CAD build for the part. Positions are in the model's coordinates, mm. A direction names the side the tool comes from. Round coordinates to 2 decimals unless told otherwise and drop trailing zeros. Answer as a JSON object with one key per item and string values.
```python
from build123d import *

# Parameters (mm, degrees)
SKETCH2_R          = 9.525
CUT_EXTRUDE1_DEPTH = 148.442344892
SKETCH3_R          = 6.35
CUT_EXTRUDE2_DEPTH = 3.81
CIRPATTERN1_COUNT  = 15
FILLET1_R          = 1.27


with BuildPart() as part:
    # Sketch1 → Revolve1 (revolve)
    with BuildSketch(Plane.XY, mode=Mode.PRIVATE) as revolve1_sk:
        with BuildLine():
            Line((0, 0), (50.8, 0))
            ThreePointArc((50.8, 0), (77.507770873, 6.756373885), (97.79, 25.4))
            Line((97.79, 25.4), (97.79, 3.81))
            Line((97.79, 3.81), (78.74, 3.81))
            Line((78.74, 3.81), (78.74, 0))
            Line((78.74, 0), (101.6, 0))
            Line((101.6, 0), (101.6, 33.077561287))
            Line((101.6, 33.077561287), (97.79, 33.077561287))
            ThreePointArc((97.79, 33.077561287), (78.479641633, 11.725205481), (50.8, 3.81))
            Line((50.8, 3.81), (0, 3.81))
            Line((0, 3.81), (0, 0))
        make_face()
    revolve(revolve1_sk.sketch.rotate(Axis((0, 0, 0), (0, 1, 0)), 90), axis=Axis((0, 0, 0), (0, 1, 0)))

    # Sketch2 → Cut-Extrude1 (cut, through all)
    with BuildSketch(Plane.XZ):
        with Locations(Location((-22.225, 0, 0), (0, 0, 270))):
            Circle(SKETCH2_R)
        with Locations(Location((22.225, 0, 0), (0, 0, 270))):
            Circle(SKETCH2_R)
    extrude(amount=-CUT_EXTRUDE1_DEPTH, mode=Mode.SUBTRACT)

    # Sketch3 → Cut-Extrude2 (cut)
    with BuildSketch(Plane.XZ):
        with Locations(Location((-88.9, 0, 0), (0, 0, 270))):
            Circle(SKETCH3_R)
    cut_extrude2 = extrude(amount=-CUT_EXTRUDE2_DEPTH, mode=Mode.SUBTRACT)

    # CirPattern1: Cut-Extrude2 ×15 about axis
    cirpattern1_axis = Axis((0, 0, 0), (0, 1, 0))
    for i in range(1, CIRPATTERN1_COUNT):
        add(cut_extrude2.rotate(cirpattern1_axis, i * 360 / CIRPATTERN1_COUNT), mode=Mode.SUBTRACT)

    # Fillet1
    fillet1_edges = [part.edges().sort_by_distance(p)[0] for p in [
        (0, 3.81, 78.74),
        (0, 3.81, 97.79),
    ]]
    fillet(fillet1_edges, radius=FILLET1_R)


solid = part.part
```
Item 1: 3-axis set-ups, long thin cutter, end or side, ignore diameter. For faces 1 (the flat face through (57, 3.81, 58)), 2 (the cylindrical face through (8.57, 1.88, -94.72)), 3 (the flat face through (-83, 33.078, 53)): which of +Z, -Z, +X, -X, +Y, -Y reach the whole face in a straight line?
Worked answers:
{"face 1": "none", "face 2": "-Y", "face 3": "+Z, -Z, +X, -X, +Y"}
Item 2: Wall check: line 1 along X through (y, z) = (19.5, -63.5); line 2 along X through (y, z) = (23, -46); line 3 along Y through (x, z) = (10, -44.5). Give the ranges that are in metal, low to high. Write a range as [from, to].
Worked answers:
{"line 1": "x = [-79.31, -74.37], [-68.42, -61.17], [61.17, 68.42], [74.37, 79.31]", "line 2": "x = [-90.59, -86.3], [-84.41, -78.88], [78.88, 84.41], [86.3, 90.59]", "line 3": "y = [0, 3.81]"}
Item 3: Drop flat-ended pins along their axis: pin 1 Ø16.5 at (x, z) = (44.45, -76.99) entering from -Y; pin 2 Ø11.5 at (x, z) = (86.96, 18.48) entering from +Y; pin 3 Ø1.5 at (x, y) = (36, 9.5) entering from +Z; pin 4 Ø10 at (y, z) = (29, 34.5) entering from -X. Give the stop position or say it passes through.
Worked answers:
{"pin 1": "stops at y = 0", "pin 2": "stops at y = 27.56", "pin 3": "stops at z = 95.29", "pin 4": "stops at x = -97.22"}
Item 4: Saw through at A-A on z = 0. State how many separate pieces and enclosed holes the cut face has, and give its area (3 significant figures).
Worked answers:
{"separate pieces": "4", "enclosed holes": "0", "area": "1,020 mm2"}
Item 5: Two-plate mould, pull along X, no slides. Class faces 4 (the cylindrical face through (-82.6, 1.9, 0.8)), 5 (the flat face through (-1, 0, -1)): released by +X, released by -X, zero draft, split by the parting line, or undercut.
Worked answers:
{"face 4": "undercut", "face 5": "zero draft"}
